The listing builds one solid part. Answer for the finished solid, in the listing's coordinates (mm). Face numbers are marked on the shaded views. A direction names the side the tool comes from. Round coordinates to 2 decimals unless told otherwise and drop trailing zeros. Write each loop counter-clockwise with the first axis right and the second up, starting at its lowest first coordinate (ties: lowest second). Pieces come first, ordered by that corner, then holes.
(1) A cutting plane is placed at B-B, the plane x = -40.5. Give the vertices of the cut face in (y, z), and give its area (3 significant figures).
(2) A cutting plane is placed at D-D, the plane y = 57.5. Give the vertices of the cut face in (x, z).
(3) Find the intervals of material crossed by probe 1 along Y at (x, z) = (-24, 1.3); probe 2 along Z at (x, y) = (36, 4); probe 3 along Y at (x, z) = (-40.5, 2.3), in increasing order.
(4) A cutting plane is placed at C-C, the plane z = 2. Give the number of separate pieces and of enclosed holes in the cut face, and give its area (3 significant figures).
(5) A cutting plane is placed at A-A, the plane x = -24. Give the vertices of the cut face in (y, z), and give its area (4 significant figures).
(6) For the marked faces 1 and 2, determine the directions among +Z, -Z, +X, -X, +Y, -Y from which every point of the face is accessible in a straight line to the end or side of a thin tool.
(7) Each of these flat-tipped pins is pushed along its axis until it touches: pin 1 Ø3 at (y, z) = (56, 1) entering from -X; pin 2 Ø12 at (y, z) = (-21.5, -8.5) entering from +X; pin 3 Ø4 at (x, y) = (-24, -36.85) entering from -Z; pin 4 Ø3 at (y, z) = (62.5, 2) entering from +X. Where does it stop, or does it pass through?
from build123d import *

# Parameters (mm, degrees)
F2_DEPTH    = 3.5
F3_R        = 1.5
F4_DEPTH    = 25
F5_W        = 15
F5_H        = 6
F6_DEPTH    = 28
F7_T1_DEPTH = 40
F8_W        = 0.6
F8_H        = 0.6
F9_DEPTH    = 0.39


# Not quite as in the source:
# - a fillet or chamfer that OpenCascade refuses, or shapes differently, is made with other operations: its cross-section is extruded or revolved along the edge and cut away or added


with BuildPart() as f2:
    # F0 (on Top) → F2 (new body)
    with BuildSketch(Plane.XY):
        Polygon((32.5, 70.6530249731), (-32.5, 70.6530249731), (-32.5, 59.4207410195), (-32.5, 48.8827627578), (-55, 25.6526721455), (-55, 5.6526721455), (-44.1446197954, -6.101506712), (-32.5, -22.3619750269), (-32.5, -39.3469750269), (32.5, -39.3469750269), (35.4572725267, -23.5087187488), (45.3055703038, -6.101506712), (55, 6.6271237275), (55, 25.6530249731), (32.5, 50.8760847151), align=None)
    extrude(amount=F2_DEPTH)

    # F3 (on face) → F4 (cut)
    with BuildSketch(Plane.XY.offset(3.5)):
        with Locations((-17.5, 65.6530249731)):
            Circle(F3_R)
        with Locations((16, 65.6530249731)):
            Circle(F3_R)
        with Locations((-40.5, 25.6526721455)):
            Circle(F3_R)
        with Locations((-40.5, 9.6526721455)):
            Circle(F3_R)
        with Locations((42, 25.6526721455)):
            Circle(F3_R)
        with Locations((42, 9.6526721455)):
            Circle(F3_R)
        with Locations((24.3198931655, -36.8469750269)):
            Circle(F3_R)
        with Locations((-24, -36.8469750269)):
            Circle(F3_R)
    extrude(amount=-F4_DEPTH, mode=Mode.SUBTRACT)

    # F5 (on face) → F6 (join)
    with BuildSketch(Plane.XY):
        with Locations((-0.6, 64.9171224535)):
            Rectangle(F5_W, F5_H)
    extrude(amount=-F6_DEPTH)

    # F7: fillet of radius 5 on 2 edges, made by hand

    # F7_s2 → F7_t1 (cut)
    with BuildSketch(Plane.YZ.offset(-20.6)):
        with BuildLine():
            ThreePointArc((61.9171224535, -23), (63.3815885475, -26.5355339059), (66.9171224535, -28))
            Line((66.9171224535, -28), (61.9171224535, -28))
            Line((61.9171224535, -28), (61.9171224535, -23))
        make_face()
        with BuildLine():
            ThreePointArc((67.9171224535, -23), (66.4526563594, -26.5355339059), (62.9171224535, -28))
            Line((62.9171224535, -28), (67.9171224535, -28))
            Line((67.9171224535, -28), (67.9171224535, -23))
        make_face()
    extrude(amount=F7_T1_DEPTH, mode=Mode.SUBTRACT)

    # F8 (on face) → F9 (join)
    with BuildSketch(Plane.XY.offset(3.5)):
        Polygon((-30.2116373062, -25.3581409693), (-30.2116373062, -25.5081409693), (-30.0116373062, -25.5081409693), (-29.9116373062, -25.5081409693), (-29.3116373062, -25.5081409693), (-29.3116373062, -25.3581409693), align=None)
        Polygon((-30.0116373062, -25.5081409693), (-30.2116373062, -25.5081409693), (-30.2116373062, -26.7081409693), (-29.9116373062, -26.7081409693), (-29.9116373062, -26.1081409693), (-29.9116373062, -25.5081409693), align=None)
        with Locations((-29.6116373062, -26.4081409693)):
            Rectangle(F8_W, F8_H)
    extrude(amount=F9_DEPTH)


solid = f2.part
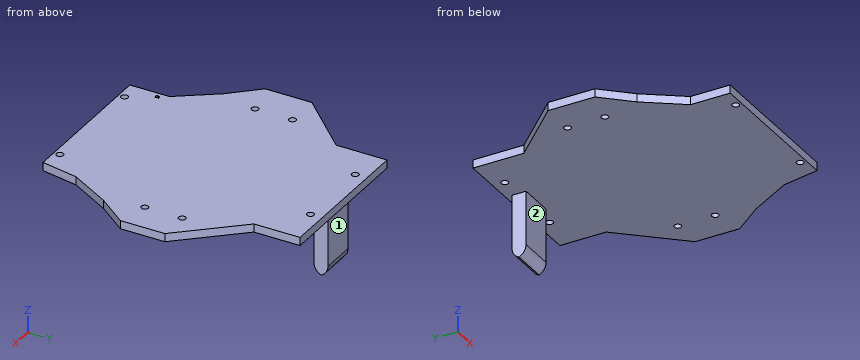
Solutions:
1. outline: (-11.19, 0) - (8.15, 0) - (8.15, 3.5) - (-11.19, 3.5) - close; (11.15, 0) - (24.15, 0) - (24.15, 3.5) - (11.15, 3.5) - close; (27.15, 0) - (40.62, 0) - (40.62, 3.5) - (27.15, 3.5) - close
1. area: 160 mm2
2. outline: (-32.5, 0) - (32.5, 0) - (32.5, 3.5) - (-32.5, 3.5) - close
3. probe 1: y = -39.35 to -38.35, -35.35 to 70.65
3. probe 2: z = 0 to 3.5
3. probe 3: y = -11.19 to 8.15, 11.15 to 24.15, 27.15 to 40.62
4. separate pieces: 1
4. enclosed holes: 8
4. area: 9,200 mm2
5. outline: (-39.35, 0) - (-38.35, 0) - (-38.35, 3.5) - (-39.35, 3.5) - close; (-35.35, 0) - (70.65, 0) - (70.65, 3.5) - (-35.35, 3.5) - close
5. area: 374.5 mm2
6. face 1: -Z, +X, -X, +Y
6. face 2: -Z, +X, -X, -Y
7. pin 1: stops at x = -32.5
7. pin 2: passes through
7. pin 3: stops at z = 0
7. pin 4: stops at x = 32.5
